Source: three-view drawing plus pictorial views. Frame: mm from the lowest corner of the part. A direction names the side the tool comes from. Give positions to 0.01 mm unless a question says otherwise; leave off trailing zeros. Write each loop counter-clockwise with the first axis right and the second up, starting at its lowest first coordinate (ties: lowest second). Pieces come first, ordered by that corner, then holes. Notation, with made-up numbers: M 89.25,89.25 L 110.25,89.25 A32 cw 110.25,123.25 Z; hole C 6.25,25 d8. An arc over 180 degrees is marked long. Return JSON: item names as keys, results as strings.
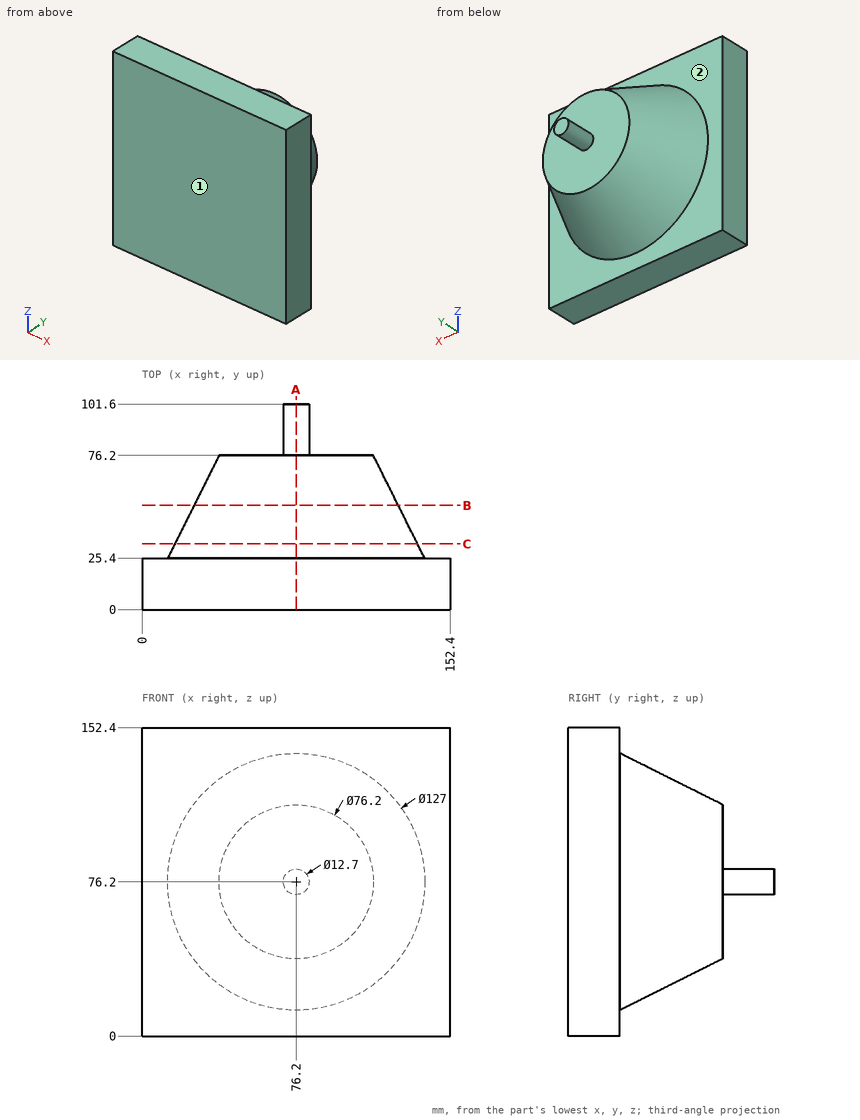
1) Set-up query: the marked faces 1 and 2. Return all of +Z, -Z, +X, -X, +Y, -Y with unobstructed straight access to the full face (end or side cutting, diameter ignored); none if empty.
Numbers:
{"face 1": "+Z, -Z, +X, -X, -Y", "face 2": "+Y"}
2) Contact query for flat-ended pins moving along their axis: pin 1 Ø2 at (y, z) = (28.5, 77) entering from -X; pin 2 Ø2 at (x, z) = (115, 43) entering from +Y; pin 3 Ø8 at (x, y) = (84.5, 86.5) entering from +Z. Output: stop coordinate, or through.
Numbers:
{"pin 1": "stops at x = 13.75", "pin 2": "stops at y = 52.27", "pin 3": "stops at z = 80.87"}
3) Line query: line 1 (Y direction, x = 45.5, z = 91); line 2 (Y direction, x = 119.5, z = 15.5); line 3 (X direction, y = 29, z = 81). Output: solid intervals per line, ascending. Write a range as [from, to].
Numbers:
{"line 1": "y = [0, 76.2]", "line 2": "y = [0, 25.4]", "line 3": "x = [14.69, 137.71]"}
4) Cut plane B-B, the plane y = 51.5. Return the cut outline in (x, z).
Numbers:
{"outline": "C 76.2,76.2 d100.9"}
5) Cut plane A-A, the plane x = 76.2. Return the cut outline in (y, z).
Numbers:
{"outline": "M 0,0 L 25.4,0 L 25.4,12.7 L 76.2,38.1 L 76.2,69.85 L 101.6,69.85 L 101.6,82.55 L 76.2,82.55 L 76.2,114.3 L 25.4,139.7 L 25.4,152.4 L 0,152.4 Z"}
6) Cut plane C-C, the plane y = 32.5. Return the cut outline in (x, z).
Numbers:
{"outline": "C 76.2,76.2 d119.9"}
